```python
from build123d import *

# Parameters (mm, degrees)
SKETCH1_R           = 5.88
BOSS_EXTRUDE1_DEPTH = 40.8
SKETCH2_R           = 9
BOSS_EXTRUDE2_DEPTH = 15
SKETCH3_R           = 5
CUT_EXTRUDE1_DEPTH  = 40
SKETCH4_W           = 8.5
SKETCH4_H           = 12
BOSS_EXTRUDE4_DEPTH = 38
SKETCH5_R           = 5.5
BOSS_EXTRUDE5_DEPTH = 25
FILLET1_R           = 5
FILLET2_R           = 5


with BuildPart() as part:
    # Sketch1 → Boss-Extrude1 (new body)
    with BuildSketch(Plane.XY):
        Circle(SKETCH1_R)
    extrude(amount=BOSS_EXTRUDE1_DEPTH)

    # Sketch2 → Boss-Extrude2 (add)
    with BuildSketch(Plane.XY.offset(40.8)):
        Circle(SKETCH2_R)
    extrude(amount=BOSS_EXTRUDE2_DEPTH)

    # Sketch3 → Cut-Extrude1 (cut)
    with BuildSketch(Plane(origin=(0, 0, 0), x_dir=(-1, 0, 0), z_dir=(0, 0, -1))):
        Circle(SKETCH3_R)
    extrude(amount=-CUT_EXTRUDE1_DEPTH, mode=Mode.SUBTRACT)

    # Sketch4 → Boss-Extrude4 (add)
    with BuildSketch(Plane(origin=(0, 0, 0), x_dir=(0, 0, -1), z_dir=(1, 0, 0))):
        with Locations((-48.767868688, -0.197628396)):
            Rectangle(SKETCH4_W, SKETCH4_H)
    extrude(amount=BOSS_EXTRUDE4_DEPTH)

    # Sketch5 → Boss-Extrude5 (add)
    with BuildSketch(Plane.XY.offset(53.017868688)):
        with Locations((32.222684983, 0)):
            Circle(SKETCH5_R)
    extrude(amount=BOSS_EXTRUDE5_DEPTH)

    # Fillet1
    fillet1_edges = [part.edges().sort_by_distance(p)[0] for p in [
        (38, 5.802371604, 48.767868688),
    ]]
    fillet(fillet1_edges, radius=FILLET1_R)

    # Fillet2
    fillet2_edges = [part.edges().sort_by_distance(p)[0] for p in [
        (38, -6.197628396, 48.767868688),
    ]]
    fillet(fillet2_edges, radius=FILLET2_R)


solid = part.part
```
Geometry check sheet. Reference: the model listing, model coordinates, mm. A direction names the side the tool comes from. Give positions to 0.01 mm unless a question says otherwise; leave off trailing zeros. Write each loop counter-clockwise with the first axis right and the second up, starting at its lowest first coordinate (ties: lowest second). Pieces come first, ordered by that corner, then holes. Notation, with made-up numbers: (53, 68) - (57, 68) arc R29 cw to (57, 102) - close; hole circle Ø8 at (19, -25.75). An arc over 180 degrees is marked (long way). Use a Markdown table: item, result.
Q1. Draft check along X on faces 6 (the face through (38, 0, 49)), 7 (the face through (0, 0, 40)), 8 (the face through (2, -6, 40.8)). Enter one of: pulls with the +X half, pulls with the -X half, needs draft (parallel to the pull), parting line crosses it, or undercut.
Computed:
| item | result |
|---|---|
| face 6 | pulls with the +X half |
| face 7 | undercut |
| face 8 | needs draft |
Q2. Set-up check for faces 1 (the face through (20, -6.198, 49)), 2 (the face through (26.728, 0.242, 65.343)), 3 (the face through (20, 5.802, 49)), 4 (the face through (0, 0, 55.8)), 5 (the face through (5.608, 1.766, 20.114)): record each of +Z, -Z, +X, -X, +Y, -Y from which the full face is reachable in a straight line by a thin tool's end or side.
Computed:
| item | result |
|---|---|
| face 1 | +Z, -Z, +X, -Y |
| face 2 | +Z |
| face 3 | +Z, -Z, +X, +Y |
| face 4 | +Z, -X, +Y, -Y |
| face 5 | -Z |
Q3. Section check C-C, the plane z = 47. Enter the section's corners in (x, y), then the cut area to 3 significant figures.
Computed:
| item | result |
|---|---|
| outline | (6.53, -6.2) - (33, -6.2) arc R5 ccw to (38, -1.2) - (38, 0.8) arc R5 ccw to (33, 5.8) - (6.88, 5.8) arc R9 ccw (long way) to start |
| area | 600 mm² |
Q4. Section check B-B, the plane x = 0. Enter the section's corners in (y, z), then the cut area to 3 significant figures.
Computed:
| item | result |
|---|---|
| outline | (-9, 40.8) - (-5.88, 40.8) - (-5.88, 0) - (-5, 0) - (-5, 40) - (5, 40) - (5, 0) - (5.88, 0) - (5.88, 40.8) - (9, 40.8) - (9, 55.8) - (-9, 55.8) - close |
| area | 350 mm² |
Q5. Section check D-D, the plane z = 32. Enter the section's corners in (x, y).
Computed:
| item | result |
|---|---|
| outline | circle Ø11.76 at (0, 0); hole circle Ø10 at (0, 0) |
Q6. Go/stop test with flat-tipped pins: P1, Ø8, axis at y = -6.5, z = 63, coming from the -X side; P2, Ø3, axis at y = -4.5, z = 21, coming from the +X side; P3, Ø12, axis at x = 14, z = 42.5, coming from the -Y side. Record where each tip stops, or that it passes through.
Computed:
| item | result |
|---|---|
| P1 | stops at x = 27.32 |
| P2 | stops at x = 5.06 |
| P3 | stops at y = -6.2 |
Q7. Thickness scan on L1, parallel to Y at x = 0, z = 25; L2, parallel to Z at x = -0.5, y = 0.5; L3, parallel to Z at x = 23.5, y = 2. Record the ranges inside material, lowest first. Write a range as [from, to].
Computed:
| item | result |
|---|---|
| L1 | y = [-5.88, -5], [5, 5.88] |
| L2 | z = [40, 55.8] |
| L3 | z = [44.52, 53.02] |
Q8. Section check A-A, the plane y = 0. Enter the section's corners in (x, z).
Computed:
| item | result |
|---|---|
| outline | (-9, 40.8) - (-5.88, 40.8) - (-5.88, 0) - (-5, 0) - (-5, 40) - (5, 40) - (5, 0) - (5.88, 0) - (5.88, 40.8) - (9, 40.8) - (9, 44.52) - (38, 44.52) - (38, 53.02) - (37.72, 53.02) - (37.72, 78.02) - (26.72, 78.02) - (26.72, 53.02) - (9, 53.02) - (9, 55.8) - (-9, 55.8) - close |
